The model under review builds one solid part; all positions refer to its coordinate system, in mm. A direction names the side the tool comes from. Coordinates: 2 decimals unless noted, no trailing zeros. Write each loop counter-clockwise with the first axis right and the second up, starting at its lowest first coordinate (ties: lowest second). Pieces come first, ordered by that corner, then holes.
1) Add section A-A, the plane y = 22.5. State the section outline as (x, z) points.
2) Add section B-B, the plane x = -30.5. State the section outline as (y, z) points, then the cut area to 3 significant figures.
3) Add section C-C, the plane z = 23.5. State the section outline as (x, y) points.
4) For P1, Ø1, axis at x = -15, y = 30, coming from the +Z side; P2, Ø11.5, axis at y = 9, z = 12.5, coming from the -X side; P3, Ø3.5, axis at x = 49.5, y = -45.5, coming from the +Z side, all flat-tipped, find the tip position at first contact; note any pin that passes through.
5) Add section D-D, the plane x = -11. State the section outline as (y, z) points.
6) Machinability: for faces 4 (the flat face through (-1, -55, 12)), 5 (the flat face through (50, -45, 2)), which of the approach directions +Z, -Z, +X, -X, +Y, -Y give a long, thin tool a straight path to every point of the face, cutting with its end or side? Answer none if there is none.
7) Mouldability with a two-part tool opening along Y and no side actions: class faces 1 (the flat face through (-60, -1, 18)), 2 (the cylindrical face through (51.343, -48.334, 3.972)), 3 (the flat face through (-1, 55, 12)) as released by +Y, released by -Y, zero draft, split by the parting line, or undercut.
8) For line 1 (X direction, y = 35, z = 2.5); line 2 (Y direction, x = 46, z = 12.5); line 3 (X direction, y = -3, z = 16.75), list the stretches that pass through material, from the lowest coordinate up.
from build123d import *

# Parameters (mm, degrees)
F0_W      = 120
F0_H      = 110
F1_DEPTH  = 25
F2_W      = 116
F2_H      = 106
F3_DEPTH  = 23
F4_R      = 3.5
F5_DEPTH  = 4
F6_R      = 1.5
F7_DEPTH  = 4
F8_R      = 1.5
F9_DEPTH  = 4
F10_R     = 1.5
F11_DEPTH = 4
F12_R     = 1.5
F13_DEPTH = 4
F14_W     = 14
F14_H     = 14
F15_DEPTH = 5
F16_W     = 12
F16_H     = 10
F16_W_2   = 30
F16_W_3   = 10
F17_DEPTH = 2
F18_DEPTH = 25
F19_DEPTH = 25
F20_DEPTH = 25
F21_DEPTH = 25
F22_W     = 1.3961357757
F22_H     = 12
F23_DEPTH = 25


with BuildPart() as f1:
    # F0 (on Top) → F1 (new body)
    with BuildSketch(Plane.XY):
        Rectangle(F0_W, F0_H)
    extrude(amount=F1_DEPTH)

    # F2 (on face) → F3 (cut)
    with BuildSketch(Plane.XY.offset(25)):
        Rectangle(F2_W, F2_H)
    extrude(amount=-F3_DEPTH, mode=Mode.SUBTRACT)

    # F4 (on face) → F5 (join)
    with BuildSketch(Plane.XY.offset(2)):
        with Locations((-50.2721771598, 34.7715031275)):
            Circle(F4_R)
        with Locations((49.7278228402, 34.7715031275)):
            Circle(F4_R)
        with Locations((49.7278228402, -45.2284968725)):
            Circle(F4_R)
        with Locations((-50.2721771598, -45.2284968725)):
            Circle(F4_R)
    extrude(amount=F5_DEPTH)

    # F6 (on face) → F7 (cut)
    with BuildSketch(Plane.XY.offset(6)):
        with Locations((-50.2721771598, 34.7715031275)):
            Circle(F6_R)
    extrude(amount=-F7_DEPTH, mode=Mode.SUBTRACT)

    # F8 (on face) → F9 (cut)
    with BuildSketch(Plane.XY.offset(6)):
        with Locations((49.7278228402, 34.7715031275)):
            Circle(F8_R)
    extrude(amount=-F9_DEPTH, mode=Mode.SUBTRACT)

    # F10 (on face) → F11 (cut)
    with BuildSketch(Plane.XY.offset(6)):
        with Locations((49.7278228402, -45.2284968725)):
            Circle(F10_R)
    extrude(amount=-F11_DEPTH, mode=Mode.SUBTRACT)

    # F12 (on face) → F13 (cut)
    with BuildSketch(Plane.XY.offset(6)):
        with Locations((-50.2721771598, -45.2284968725)):
            Circle(F12_R)
    extrude(amount=-F13_DEPTH, mode=Mode.SUBTRACT)

    # F14 (on face) → F15 (cut)
    with BuildSketch(Plane.XZ.offset(55)):
        with Locations((-33.3, 12)):
            Rectangle(F14_W, F14_H)
    extrude(amount=-F15_DEPTH, mode=Mode.SUBTRACT)

    # F16 (on face) → F17 (cut)
    with BuildSketch(Plane(origin=(-60, 0, 0), x_dir=(0, -1, 0), z_dir=(-1, 0, 0))):
        with Locations((35, 10)):
            Rectangle(F16_W, F16_H)
        with Locations((13, 10)):
            Rectangle(F16_W, F16_H)
        with Locations((-13, 10)):
            Rectangle(F16_W_2, F16_H)
        with Locations((-43, 10)):
            Rectangle(F16_W_3, F16_H)
    extrude(amount=-F17_DEPTH, mode=Mode.SUBTRACT)

    # F4 (on face) → F18 (cut)
    with BuildSketch(Plane.XY.offset(2)):
        with BuildLine():
            Line((-45.2721779048, 7.7715031275), (-0.2721771598, 7.7715031275))
            Line((-0.2721771598, 7.7715031275), (-0.2721771598, 17.7715031275))
            Line((-0.2721771598, 17.7715031275), (-45.2721779048, 17.7715031275))
            ThreePointArc((-45.2721779048, 17.7715031275), (-48.8077118108, 16.3070370335), (-50.2721779048, 12.7715031275))
            ThreePointArc((-50.2721779048, 12.7715031275), (-48.8077118108, 9.2359692216), (-45.2721779048, 7.7715031275))
        make_face()
        with BuildLine():
            Line((-0.2721771598, 17.7715031275), (-0.2721771598, 7.7715031275))
            Line((-0.2721771598, 7.7715031275), (44.7278220952, 7.7715031275))
            ThreePointArc((44.7278220952, 7.7715031275), (48.2633560011, 9.2359692216), (49.7278220952, 12.7715031275))
            ThreePointArc((49.7278220952, 12.7715031275), (48.2633560011, 16.3070370335), (44.7278220952, 17.7715031275))
            Line((44.7278220952, 17.7715031275), (-0.2721771598, 17.7715031275))
        make_face()
    extrude(amount=-F18_DEPTH, mode=Mode.SUBTRACT)

    # F4 (on face) → F19 (cut)
    with BuildSketch(Plane.XY.offset(2)):
        with BuildLine():
            Line((-0.2721771598, -18.2284968725), (-0.2721771598, -28.2284968725))
            Line((-0.2721771598, -28.2284968725), (44.7278220952, -28.2284968725))
            ThreePointArc((44.7278220952, -28.2284968725), (48.2633560011, -26.7640307784), (49.7278220952, -23.2284968725))
            ThreePointArc((49.7278220952, -23.2284968725), (48.2633560011, -19.6929629665), (44.7278220952, -18.2284968725))
            Line((44.7278220952, -18.2284968725), (-0.2721771598, -18.2284968725))
        make_face()
        with BuildLine():
            Line((49.7278228402, -5.2284968725), (-0.2721771598, -5.2284968725))
            Line((-0.2721771598, -5.2284968725), (-0.2721771598, -10.2284968725))
            Line((-0.2721771598, -10.2284968725), (44.7278228402, -10.2284968725))
            ThreePointArc((44.7278228402, -10.2284968725), (48.2633567461, -8.7640307784), (49.7278228402, -5.2284968725))
        make_face()
        with BuildLine():
            ThreePointArc((-45.2721771598, -0.2284968725), (-48.8077110657, -1.6929629665), (-50.2721771598, -5.2284968725))
            Line((-50.2721771598, -5.2284968725), (-0.2721771598, -5.2284968725))
            Line((-0.2721771598, -5.2284968725), (-0.2721771598, -0.2284968725))
            Line((-0.2721771598, -0.2284968725), (-45.2721771598, -0.2284968725))
        make_face()
        with BuildLine():
            Line((-0.2721771598, -5.2284968725), (-50.2721771598, -5.2284968725))
            ThreePointArc((-50.2721771598, -5.2284968725), (-48.8077110657, -8.7640307784), (-45.2721771598, -10.2284968725))
            Line((-45.2721771598, -10.2284968725), (-0.2721771598, -10.2284968725))
            Line((-0.2721771598, -10.2284968725), (-0.2721771598, -5.2284968725))
        make_face()
        with BuildLine():
            Line((-45.2721779048, -28.2284968725), (-0.2721771598, -28.2284968725))
            Line((-0.2721771598, -28.2284968725), (-0.2721771598, -18.2284968725))
            Line((-0.2721771598, -18.2284968725), (-45.2721779048, -18.2284968725))
            ThreePointArc((-45.2721779048, -18.2284968725), (-48.8077118108, -19.6929629665), (-50.2721779048, -23.2284968725))
            ThreePointArc((-50.2721779048, -23.2284968725), (-48.8077118108, -26.7640307784), (-45.2721779048, -28.2284968725))
        make_face()
        with BuildLine():
            Line((-0.2721771598, -0.2284968725), (-0.2721771598, -5.2284968725))
            Line((-0.2721771598, -5.2284968725), (49.7278228402, -5.2284968725))
            ThreePointArc((49.7278228402, -5.2284968725), (48.2633567461, -1.6929629665), (44.7278228402, -0.2284968725))
            Line((44.7278228402, -0.2284968725), (-0.2721771598, -0.2284968725))
        make_face()
    extrude(amount=-F19_DEPTH, mode=Mode.SUBTRACT)

    # F4 (on face) → F20 (cut)
    with BuildSketch(Plane.XY.offset(2)):
        with BuildLine():
            ThreePointArc((2.4778228402, 32.4033908546), (1.6723664885, 34.3479345029), (-0.2721771598, 35.1533908546))
            Line((-0.2721771598, 35.1533908546), (-0.2721771598, 29.6533908546))
            ThreePointArc((-0.2721771598, 29.6533908546), (1.6723664885, 30.4588472063), (2.4778228402, 32.4033908546))
        make_face()
        with BuildLine():
            Line((-0.2721771598, 29.6533908546), (-0.2721771598, 35.1533908546))
            ThreePointArc((-0.2721771598, 35.1533908546), (-3.0221771598, 32.4033908546), (-0.2721771598, 29.6533908546))
        make_face()
    extrude(amount=-F20_DEPTH, mode=Mode.SUBTRACT)

    # F4 (on face) → F21 (cut)
    with BuildSketch(Plane.XY.offset(2)):
        with BuildLine():
            Line((-0.2721771598, -37.3684372604), (-0.2721771598, -42.8684372604))
            ThreePointArc((-0.2721771598, -42.8684372604), (1.6723664885, -42.0629809087), (2.4778228402, -40.1184372604))
            ThreePointArc((2.4778228402, -40.1184372604), (1.6723664885, -38.1738936121), (-0.2721771598, -37.3684372604))
        make_face()
        with BuildLine():
            ThreePointArc((-0.2721771598, -37.3684372604), (-3.0221771598, -40.1184372604), (-0.2721771598, -42.8684372604))
            Line((-0.2721771598, -42.8684372604), (-0.2721771598, -37.3684372604))
        make_face()
    extrude(amount=-F21_DEPTH, mode=Mode.SUBTRACT)

    # F22 (on face) → F23 (cut)
    with BuildSketch(Plane.YZ.offset(60)):
        with Locations((8.0433619022, 11)):
            Rectangle(F22_W, F22_H)
        with Locations((3.0433619022, 11)):
            Rectangle(F22_W, F22_H)
        with Locations((-1.9566380978, 11)):
            Rectangle(F22_W, F22_H)
        with Locations((-6.9566380978, 11)):
            Rectangle(F22_W, F22_H)
        with Locations((-11.9566380978, 11)):
            Rectangle(F22_W, F22_H)
        with Locations((-16.9566380978, 11)):
            Rectangle(F22_W, F22_H)
        with Locations((-21.9566380978, 11)):
            Rectangle(F22_W, F22_H)
        with Locations((-26.9566380978, 11)):
            Rectangle(F22_W, F22_H)
        with Locations((-31.9566380978, 11)):
            Rectangle(F22_W, F22_H)
        with Locations((-36.9566380978, 11)):
            Rectangle(F22_W, F22_H)
    extrude(amount=-F23_DEPTH, mode=Mode.SUBTRACT)


solid = f1.part
Geometry results:
1. outline: (-60, 0) - (60, 0) - (60, 25) - (58, 25) - (58, 2) - (-58, 2) - (-58, 5) - (-60, 5) - close; (-60, 15) - (-58, 15) - (-58, 25) - (-60, 25) - close
2. outline: (-55, 0) - (-28.23, 0) - (-28.23, 2) - (-53, 2) - (-53, 5) - (-55, 5) - close; (-55, 19) - (-53, 19) - (-53, 25) - (-55, 25) - close; (-18.23, 0) - (-10.23, 0) - (-10.23, 2) - (-18.23, 2) - close; (-0.23, 0) - (7.77, 0) - (7.77, 2) - (-0.23, 2) - close; (17.77, 0) - (55, 0) - (55, 25) - (53, 25) - (53, 2) - (17.77, 2) - close
2. area: 224 mm2
3. outline: (-60, -55) - (60, -55) - (60, 55) - (-60, 55) - close; hole (-58, -53) - (58, -53) - (58, 53) - (-58, 53) - close
4. P1: stops at z = 2
4. P2: stops at x = -60
4. P3: stops at z = 6
5. outline: (-55, 0) - (-28.23, 0) - (-28.23, 2) - (-53, 2) - (-53, 25) - (-55, 25) - close; (-18.23, 0) - (-10.23, 0) - (-10.23, 2) - (-18.23, 2) - close; (-0.23, 0) - (7.77, 0) - (7.77, 2) - (-0.23, 2) - close; (17.77, 0) - (55, 0) - (55, 25) - (53, 25) - (53, 2) - (17.77, 2) - close
6. face 4: +Z, -Z, +X, -X, -Y
6. face 5: +Z
7. face 1: zero draft
7. face 2: undercut
7. face 3: released by +Y
8. line 1: x = -60 to -58, -53.76 to -51.75, -48.79 to -46.78, 46.24 to 48.25, 51.21 to 53.22, 58 to 60
8. line 2: y = -55 to -53, 53 to 55
8. line 3: x = -60 to -58, 58 to 60
